Work out the finished part from the listing and answer in its coordinate system (mm). Give positions to 0.01 mm unless a question says otherwise; leave off trailing zeros. Write each loop counter-clockwise with the first axis right and the second up, starting at its lowest first coordinate (ties: lowest second). Pieces come first, ordered by that corner, then holes.
1) Given pin 1 Ø1.5 at (x, y) = (1.5, 31.5) entering from -Z; pin 2 Ø1.5 at (x, y) = (2.5, 20.5) entering from +Z, each flat-ended and moving along its own axis, determine where each tip first touches the part or whether it passes through.
2) Find section B-B (x = 1.1). Determine the outline of the cut face in (y, z).
3) Straight lines are drawn through the part: probe 1 along Y at (x, z) = (1.6, -7.94); probe 2 along Z at (x, y) = (1.7, 17.5); probe 3 along Y at (x, z) = (0.35, 10.5). For each, find the intervals that lie inside material, in ascending order.
4) Find section A-A (y = 45.94). Determine the outline of the cut face in (x, z).
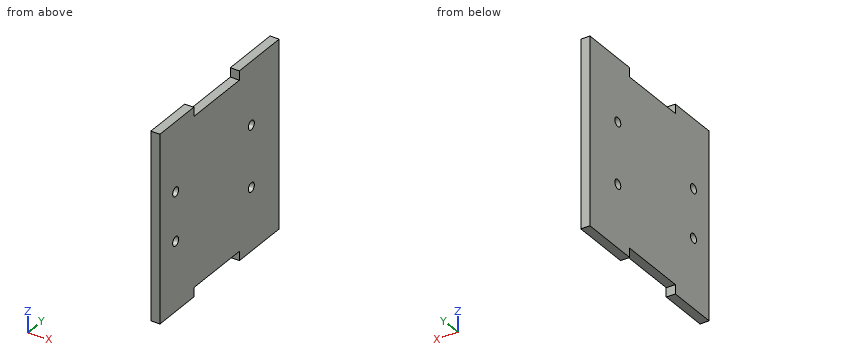
```python
from build123d import *

# Parameters (mm, degrees)
BOSS_EXTRUDE1_DEPTH   = 3
CROQUIS1_R            = 1.5
CORTAR_EXTRUIR1_DEPTH = 10


with BuildPart() as part:
    # Sketch1 → Boss-Extrude1 (new body)
    with BuildSketch(Plane(origin=(0, 0, 0), x_dir=(0, 0, -1), z_dir=(1, 0, 0))):
        Polygon((-27.5, 0), (27.5, 0), (30.5, 0), (30.5, 17), (27.5, 17), (27.5, 39.94), (30.5, 39.94), (30.5, 59.94), (27.5, 59.94), (-27.5, 59.94), (-30.5, 59.94), (-30.5, 39.94), (-27.5, 39.94), (-27.5, 17), (-30.5, 17), (-30.5, 0), align=None)
    extrude(amount=BOSS_EXTRUDE1_DEPTH)

    # Croquis1 → Cortar-Extruir1 (cut)
    with BuildSketch(Plane.ZY):
        with Locations((-7.94, 7.91)):
            Circle(CROQUIS1_R)
        with Locations(Location((7.94, 7.91, 0), (0, 0, 180))):
            Circle(CROQUIS1_R)
        with Locations((-10, 45.94)):
            Circle(CROQUIS1_R)
        with Locations(Location((10, 45.94, 0), (0, 0, 180))):
            Circle(CROQUIS1_R)
    extrude(amount=-CORTAR_EXTRUIR1_DEPTH, mode=Mode.SUBTRACT)


solid = part.part
```
Results:
1. pin 1: stops at z = -27.5
1. pin 2: stops at z = 27.5
2. outline: (0, -30.5) - (17, -30.5) - (17, -27.5) - (39.94, -27.5) - (39.94, -30.5) - (59.94, -30.5) - (59.94, 30.5) - (39.94, 30.5) - (39.94, 27.5) - (17, 27.5) - (17, 30.5) - (0, 30.5) - close; hole circle Ø3 at (7.91, -7.94); hole circle Ø3 at (7.91, 7.94); hole circle Ø3 at (45.94, -10); hole circle Ø3 at (45.94, 10)
3. probe 1: y = 0 to 6.41, 9.41 to 59.94
3. probe 2: z = -27.5 to 27.5
3. probe 3: y = 0 to 44.53, 47.35 to 59.94
4. outline: (0, -30.5) - (3, -30.5) - (3, -11.5) - (0, -11.5) - close; (0, -8.5) - (3, -8.5) - (3, 8.5) - (0, 8.5) - close; (0, 11.5) - (3, 11.5) - (3, 30.5) - (0, 30.5) - close
